```python
from build123d import *

# Parameters (mm, degrees)
EXTRUDE_1_REACH          = 103.119
CUT_EXTRUDE_2_DEPTH      = 102.118742254
PATTERN_CIRCULAR_2_COUNT = 8
CUT_EXTRUDE_3_DEPTH      = 102.118742254


with BuildPart() as part:
    # Sketch 7 → Loft 4 section 0
    with BuildSketch(Plane(origin=(0, 55, 0), x_dir=(1, 0, 0), z_dir=(0, 1, 0))):
        with BuildLine():
            Line((0, 32.471766009), (-22.961005942, 22.961005942))
            Line((-22.961005942, 22.961005942), (-32.471766009, 0))
            Line((-32.471766009, 0), (-22.961005942, -22.961005942))
            Line((-22.961005942, -22.961005942), (0, -32.471766009))
            Line((0, -32.471766009), (22.961005942, -22.961005942))
            Line((22.961005942, -22.961005942), (32.471766009, 0))
            Line((32.471766009, 0), (22.961005942, 22.961005942))
            Line((22.961005942, 22.961005942), (0, 32.471766009))
        make_face()
    # Sketch 1 → Loft 4 section 1
    with BuildSketch(Plane(origin=(0, 0, 0), x_dir=(1, 0, 0), z_dir=(0, 1, 0))):
        with BuildLine():
            Line((0, 60), (-42.426406871, 42.426406871))
            Line((-42.426406871, 42.426406871), (-60, 0))
            Line((-60, 0), (-42.426406871, -42.426406871))
            Line((-42.426406871, -42.426406871), (0, -60))
            Line((0, -60), (42.426406871, -42.426406871))
            Line((42.426406871, -42.426406871), (60, 0))
            Line((60, 0), (42.426406871, 42.426406871))
            Line((42.426406871, 42.426406871), (0, 60))
        make_face()
    loft()

    # Sketch 9 → Extrude 1 (add, up to next)
    with BuildSketch(Plane(origin=(0, 55, 0), x_dir=(1, 0, 0), z_dir=(0, 1, 0)), mode=Mode.PRIVATE) as extrude_1_sk1:
        Polygon((27.716385975, 11.480502971), (60, 0), (27.716385975, -11.480502971), align=None)
    extrude_1_tool1 = extrude(extrude_1_sk1.sketch, amount=-EXTRUDE_1_REACH, mode=Mode.PRIVATE) - part.part
    extrude_1 = extrude_1_tool1.solids().sort_by_distance((38.477591, 55, 0))[0]
    add(extrude_1)

    # Sketch 10 → Cut-Extrude 2 (cut, symmetric)
    with BuildSketch(Plane.XY):
        Polygon((-175.786069036, 212.589586203), (27.716385975, 55), (60, 30), (263.502455012, -127.589586203), (578.681627419, 279.41532382), (139.39310337, 619.594496227), align=None)
    cut_extrude_2 = extrude(amount=CUT_EXTRUDE_2_DEPTH, both=True, mode=Mode.SUBTRACT)

    # Pattern Circular 2: Extrude 1, Cut-Extrude 2 ×8 about axis
    pattern_circular_2_axis = Axis((0, 0, 0), (0, 1, 0))
    add([extrude_1.rotate(pattern_circular_2_axis, i * 360 / PATTERN_CIRCULAR_2_COUNT) for i in range(1, PATTERN_CIRCULAR_2_COUNT)])
    add([cut_extrude_2.rotate(pattern_circular_2_axis, i * 360 / PATTERN_CIRCULAR_2_COUNT) for i in range(1, PATTERN_CIRCULAR_2_COUNT)], mode=Mode.SUBTRACT)

    # Sketch 12 → Cut-Extrude 3 (cut, through all)
    with BuildSketch(Plane(origin=(0, 55, 0), x_dir=(1, 0, 0), z_dir=(0, 1, 0))):
        Polygon((22.716385975, -9.409435159), (22.716385975, 9.409435159), (9.409435159, 22.716385975), (-9.409435159, 22.716385975), (-22.716385975, 9.409435159), (-22.716385975, -9.409435159), (-9.409435159, -22.716385975), (9.409435159, -22.716385975), align=None)
    extrude(amount=-CUT_EXTRUDE_3_DEPTH, mode=Mode.SUBTRACT)


solid = part.part
```
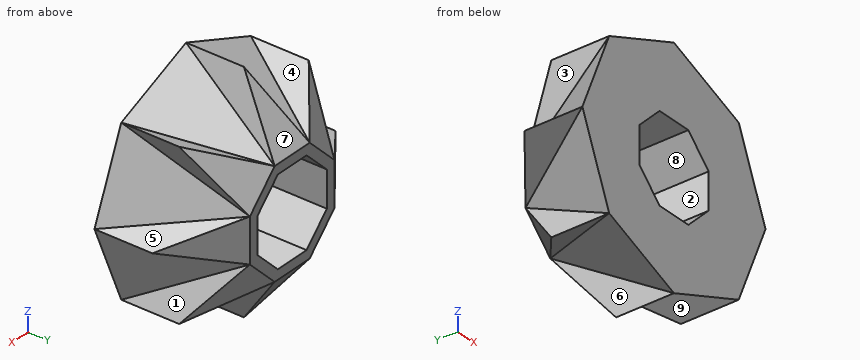
Verification items for the finished model (mm, model axes). Face numbers are marked on the shaded views. A direction names the side the tool comes from. Round coordinates to 2 decimals unless told otherwise and drop trailing zeros. Answer as a JSON object with one key per item and string values. Group by question number.
Q1. Thickness scan on line 1 (Z direction, x = -41.5, y = 18); line 2 (Z direction, x = 19, y = 50.5); line 3 (X direction, y = 28.5, z = -6). Record the ranges inside material, lowest first.
Q2. Tool access check on the marked faces 1, 2, 3, 4 and 5. Record the directions out of +Z, -Z, +X, -X, +Y, -Y that give a thin tool (end or side, any length) a straight path to the whole face; none if there is none.
Q3. Go/stop test with flat-tipped pins: pin 1 Ø4 at (x, z) = (6, -38.5) entering from -Y; pin 2 Ø3 at (x, y) = (-26.5, 45) entering from -Z; pin 3 Ø10 at (x, y) = (23.5, 28) entering from -Z; pin 4 Ø5 at (y, z) = (5.5, -26) entering from -X. Record where each tip stops, or that it passes through.
Q4. Mould release check, pull along X, two halves, no side actions. Record for the marked faces 6, 7, 8 and 9: released by +X, released by -X, zero draft, split by the parting line, or undercut.
Found:
{
 "1": {"line 1": "z = -41.99 to -40.48, -22.91 to 22.91, 40.48 to 41.99", "line 2": "z = -28.41 to -13.13, 13.13 to 28.41", "line 3": "x = -43.25 to -22.72, 22.72 to 43.25"},
 "2": {"face 1": "+X, +Y", "face 2": "+Y, -Y", "face 3": "-X, +Y", "face 4": "+Z, +Y", "face 5": "+Z, +X, +Y"},
 "3": {"pin 1": "stops at y = 0", "pin 2": "stops at z = -34.08", "pin 3": "stops at z = -39.5", "pin 4": "stops at x = -48.1"},
 "4": {"face 6": "released by -X", "face 7": "zero draft", "face 8": "undercut", "face 9": "undercut"}
}
